Build history of the part. All positions in model axes, mm. A direction names the side the tool comes from. Round coordinates to 2 decimals unless told otherwise and drop trailing zeros. Write each loop counter-clockwise with the first axis right and the second up, starting at its lowest first coordinate (ties: lowest second). Pieces come first, ordered by that corner, then holes.
Item 1: Band-saw the part on A-A, the plane y = 0. Write the cut outline in (x, z), then the cut area to 3 significant figures.
Item 2: Band-saw the part on C-C, the plane y = -3.5. Write the cut outline in (x, z), then the cut area to 3 significant figures.
Item 3: Band-saw the part on B-B, the plane x = -6. Write the cut outline in (y, z).
Item 4: Drop flat-ended pins along their axis: pin 1 Ø0.9 at (x, y) = (16.5, -8.5) entering from +Z; pin 2 Ø2.5 at (y, z) = (2, 1.5) entering from -X. Give the stop position or say it passes through.
Item 5: 3-axis set-ups, long thin cutter, end or side, ignore diameter. For faces 1 (the flat face through (-16, -9, 1)), 2 (the flat face through (0, 0, 2)), 3 (the flat face through (9, 0, 1)), 4 (the flat face through (20, 0, 1)), 5 (the cylindrical face through (-18.859, -11.297, 1.521)): which of +Z, -Z, +X, -X, +Y, -Y reach the whole face in a straight line?
Item 6: Band-saw the part on D-D, the plane x = 8. Write the cut outline in (y, z).
Item 7: Wall check: probe 1 along Y at (x, z) = (-16, 4); probe 2 along X at (y, z) = (6, 0.5); probe 3 along X at (y, z) = (-1, 2.85). Give the ranges that are in metal, low to high.
Item 8: Mould opens along Y. For faces 6 (the cylindrical face through (-18.859, 11.297, 1.521)), 7 (the cylindrical face through (8.43, 7.4, 1.01)), 8 (the flat face through (-23, 0, 3)) say: +Y half, -Y half, draft (parallel to the pull), parting line (faces both ways), or undercut.
```python
from build123d import *

# Parameters (mm, degrees)
F0_W      = 40
F0_H      = 25
F1_DEPTH  = 3
F2_R      = 4
F3_W      = 52
F3_H      = 25
F4_DEPTH  = 2
F5_R      = 3
F6_R      = 1.5
F7_DEPTH  = 25
F8_R      = 1.5
F9_DEPTH  = 4
F10_W     = 24
F10_H     = 25
F11_DEPTH = 3
F12_W     = 4
F12_H     = 16
F12_R     = 4
F13_DEPTH = 25
F14_R     = 1.99999


# Not quite as in the source:
# - a fillet or chamfer is up to 0.001 mm smaller than in the source, because OpenCascade refuses the exact size


with BuildPart() as f1:
    # F0 (on Top) → F1 (new body)
    with BuildSketch(Plane.XY):
        Rectangle(F0_W, F0_H)
    extrude(amount=F1_DEPTH)

    # F2
    f2_edges = [f1.edges().sort_by_distance(p)[0] for p in [
        (-20, -12.5, 1.5),
        (-20, 12.5, 1.5),
        (20, -12.5, 1.5),
        (20, 12.5, 1.5),
    ]]
    fillet(f2_edges, radius=F2_R)

    # F3 (on face) → F4 (join)
    with BuildSketch(Plane.XY.offset(3)):
        Rectangle(F3_W, F3_H)
    extrude(amount=F4_DEPTH)

    # F5
    f5_edges = [f1.edges().sort_by_distance(p)[0] for p in [
        (26, 12.5, 4),
        (26, -12.5, 4),
        (-26, -12.5, 4),
        (-26, 12.5, 4),
    ]]
    fillet(f5_edges, radius=F5_R)

    # F6 (on Top) → F7 (cut)
    with BuildSketch(Plane.XY):
        with Locations((23, 9)):
            Circle(F6_R)
        with Locations((23, -9)):
            Circle(F6_R)
        with Locations((-23, -9)):
            Circle(F6_R)
        with Locations((-23, 9)):
            Circle(F6_R)
    extrude(amount=F7_DEPTH, mode=Mode.SUBTRACT)

    # F8 (on face) → F9 (cut)
    with BuildSketch(Plane.XY.offset(5)):
        with Locations((16, -9)):
            Circle(F8_R)
        with Locations((-16, -9)):
            Circle(F8_R)
        with Locations((-16, 9)):
            Circle(F8_R)
        with Locations((16, 9)):
            Circle(F8_R)
    extrude(amount=-F9_DEPTH, mode=Mode.SUBTRACT)

    # F10 (on face) → F11 (cut)
    with BuildSketch(Plane.XY.offset(5)):
        Rectangle(F10_W, F10_H)
    extrude(amount=-F11_DEPTH, mode=Mode.SUBTRACT)

    # F12 (on face) → F13 (cut)
    with BuildSketch(Plane(origin=(0, 0, 0), x_dir=(1, 0, 0), z_dir=(0, 0, -1))):
        with Locations((7, 0)):
            Rectangle(F12_W, F12_H)
        with Locations((-6, -6)):
            Circle(F12_R)
        with Locations((-6, 6)):
            Circle(F12_R)
    extrude(amount=-F13_DEPTH, mode=Mode.SUBTRACT)

    # F14 (radius 2 in the source; OpenCascade refuses exactly that, so slightly less here)
    f14_edges = [f1.edges().sort_by_distance(p)[0] for p in [
        (9, 8, 1),
        (5, 8, 1),
        (9, -8, 1),
        (5, -8, 1),
    ]]
    fillet(f14_edges, radius=F14_R)


solid = f1.part
```
Results:
1. outline: (-26, 3) - (-20, 3) - (-20, 0) - (5, 0) - (5, 2) - (-12, 2) - (-12, 5) - (-26, 5) - close; (9, 0) - (20, 0) - (20, 3) - (26, 3) - (26, 5) - (12, 5) - (12, 2) - (9, 2) - close
1. area: 144 mm2
2. outline: (-26, 3) - (-20, 3) - (-20, 0) - (-9.12, 0) - (-9.12, 2) - (-12, 2) - (-12, 5) - (-26, 5) - close; (-2.88, 0) - (5, 0) - (5, 2) - (-2.88, 2) - close; (9, 0) - (20, 0) - (20, 3) - (26, 3) - (26, 5) - (12, 5) - (12, 2) - (9, 2) - close
2. area: 132 mm2
3. outline: (-12.5, 0) - (-10, 0) - (-10, 2) - (-12.5, 2) - close; (-2, 0) - (2, 0) - (2, 2) - (-2, 2) - close; (10, 0) - (12.5, 0) - (12.5, 2) - (10, 2) - close
4. pin 1: stops at z = 1
4. pin 2: stops at x = -20
5. face 1: +Z
5. face 2: +Z, +Y, -Y
5. face 3: +Z, -Z
5. face 4: -Z, +X, +Y, -Y
5. face 5: -Z, -X, -Y
6. outline: (-12.5, 0) - (-7.73, 0) - (-7.73, 2) - (-12.5, 2) - close; (7.73, 0) - (12.5, 0) - (12.5, 2) - (7.73, 2) - close
7. probe 1: y = -12.5 to -10.5, -7.5 to 7.5, 10.5 to 12.5
7. probe 2: x = -20 to -10, -2 to 5, 9 to 20
7. probe 3: x = -20 to -12, 12 to 20
8. face 6: +Y half
8. face 7: undercut
8. face 8: draft
